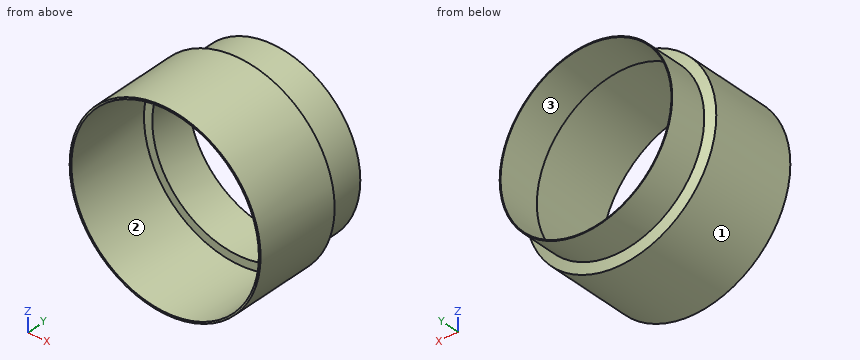
```python
from build123d import *

# Parameters (mm, degrees)
SKETCH1_R           = 40.7
SKETCH1_R_2         = 40.3
BOSS_EXTRUDE1_DEPTH = 20
SKETCH2_R           = 45.025
SKETCH2_R_2         = 44.225
BOSS_EXTRUDE2_DEPTH = 40
SKETCH3_R           = 45.025
SKETCH3_R_2         = 40.7
BOSS_EXTRUDE3_DEPTH = 0.8
CHAMFER1_SIZE       = 4.3
CHAMFER1_SIZE2      = 1.565072007


with BuildPart() as part:
    # Sketch1 → Boss-Extrude1 (new body)
    with BuildSketch(Plane(origin=(0, 0, 0), x_dir=(1, 0, 0), z_dir=(0, 1, 0))):
        Circle(SKETCH1_R)
        Circle(SKETCH1_R_2, mode=Mode.SUBTRACT)
    extrude(amount=BOSS_EXTRUDE1_DEPTH)



with BuildPart() as body_2:
    # Sketch2 → Boss-Extrude2 (new body)
    with BuildSketch(Plane.XZ):
        Circle(SKETCH2_R)
        Circle(SKETCH2_R_2, mode=Mode.SUBTRACT)
    extrude(amount=BOSS_EXTRUDE2_DEPTH)


with BuildPart() as part_1:
    add(part.part)

    add(body_2.part)  # Boss-Extrude3 merges body 2
    # Sketch3 → Boss-Extrude3 (add)
    with BuildSketch(Plane(origin=(0, 0, 0), x_dir=(1, 0, 0), z_dir=(0, 1, 0))):
        Circle(SKETCH3_R)
        Circle(SKETCH3_R_2, mode=Mode.SUBTRACT)
    extrude(amount=BOSS_EXTRUDE3_DEPTH)

    # Chamfer1
    chamfer1_edges = [part_1.edges().sort_by_distance(p)[0] for p in [
        (-40.7, 0.8, 0),
    ]]
    chamfer1_side = [part_1.faces().sort_by_distance(p)[0] for p in [
        (-43.751500687, 0.8, 0),
    ]]
    chamfer(chamfer1_edges, length=CHAMFER1_SIZE, length2=CHAMFER1_SIZE2, reference=chamfer1_side[0])


solid = part_1.part
```
Work out the finished part from the listing and answer in its coordinate system (mm). Face numbers are marked on the shaded views. Coordinates: 2 decimals unless noted, no trailing zeros. Loops run counter-clockwise (first coordinate to the right, second up) from the corner with the lowest first, then second, coordinate; pieces in that order, holes last.
1) For a pull along Z with two mould halves and no side action, classify the marked faces 1, 2 and 3 as +Z half, -Z half, draft (parallel to the pull), parting line (faces both ways), or undercut.
Results:
face 1: parting line
face 2: undercut
face 3: undercut
2) Consider probe 1 along Z at (x, y) = (0, 5); probe 2 along Z at (x, y) = (-1, -20.5). Determine where each line is inside the solid, lowest interval first.
Results:
probe 1: z = -40.7 to -40.3, 40.3 to 40.7
probe 2: z = -45.01 to -44.21, 44.21 to 45.01
3) Section C-C (y = 7.5) is taken. Give the vertices of the cut face in (x, z), plus the area to 3 significant figures.
Results:
outline: circle Ø81.4 at (0, 0); hole circle Ø80.6 at (0, 0)
area: 102 mm2
4) Section D-D (y = -3) is taken. Give the vertices of the cut face in (x, z) (3 decimals), plus the area to 3 significant figures.
Results:
outline: circle Ø90.05 at (0, 0); hole circle Ø88.45 at (0, 0)
area: 224 mm2
5) Section A-A (x = 0) is taken. Give the vertices of the cut face in (y, z) (3 decimals), plus the area to 4 significant figures.
Results:
outline: (-40, -45.025) - (0.8, -45.025) - (0.8, -45) - (2.365, -40.7) - (20, -40.7) - (20, -40.3) - (0, -40.3) - (0, -44.225) - (-40, -44.225) - close; (-40, 44.225) - (0, 44.225) - (0, 40.3) - (20, 40.3) - (20, 40.7) - (2.365, 40.7) - (0.8, 45) - (0.8, 45.025) - (-40, 45.025) - close
area: 93.65 mm2
6) Section B-B (z = 0) is taken. Give the vertices of the cut face in (x, y) (3 decimals), plus the area to 4 significant figures.
Results:
outline: (-45.025, -40) - (-44.225, -40) - (-44.225, 0) - (-40.3, 0) - (-40.3, 20) - (-40.7, 20) - (-40.7, 2.365) - (-45, 0.8) - (-45.025, 0.8) - close; (40.3, 0) - (44.225, 0) - (44.225, -40) - (45.025, -40) - (45.025, 0.8) - (45, 0.8) - (40.7, 2.365) - (40.7, 20) - (40.3, 20) - close
area: 93.65 mm2
7) Flat-ended cylindrical pins translate along their axes: pin 1 (5 mm diameter, centred on x = -5, y = 9.5, fed in from +Z); pin 2 (8 mm diameter, centred on y = -12.5, z = -13, fed in from +X); pin 3 (12 mm diameter, centred on y = -13, z = -26, fed in from +X); pin 4 (12 mm diameter, centred on x = -25, z = -32.5, fed in from -Y). Find the tip coordinate at first contact, or state that the pin passes through.
Results:
pin 1: stops at z = 40.62
pin 2: stops at x = 44.12
pin 3: stops at x = 40.34
pin 4: stops at y = -40
